Autodesk Inventor part; units mm, degrees
ref_plane "YZ Plane" through (0, 0, 0) normal (1, 0, 0) x (0, 1, 0)
ref_plane "XZ Plane" through (0, 0, 0) normal (0, 1, 0) x (-1, 0, 0)
ref_plane "XY Plane" through (0, 0, 0) normal (0, 0, 1) x (1, 0, 0)
sketch "Sketch1" plane through (0, 0, 0) normal (0, 0, 1) x (1, 0, 0)
  line L0 (0, 0) -> (33, 0)
  line L1 (33, 0) -> (33, 28)
  line L2 (33, 28) -> (0, 28)
  line L3 (0, 28) -> (0, 0)
  circle A0 centre (16.5, 14) radius 4
  circle A1 centre (16.5, 23.5) radius 1.5
  circle A2 centre (9, 5) radius 1.5
  circle A3 centre (24, 5) radius 1.5
  dimension "d0" = 33
  dimension "d1" = 28
  dimension "d2" = 8
  dimension "d3" = 14
  dimension "d4" = 16.5
  dimension "d5" = 3
  dimension "d6" = 3
  dimension "d7" = 3
  dimension "d8" = 4.5
  dimension "d9" = 0
  dimension "d10" = 15
  dimension "d11" = 5
  dimension "d12" = 9
  dimension "d13" = 5
extrude "Extrusion1" add sketch "Sketch1" along normal blind 3
sketch "Sketch2" plane through (0, 0, 3) normal (0, 0, 1) x (1, 0, 0)
  circle A0 centre (16.5, 14) radius 4
  circle A1 centre (16.5, 14) radius 5.5
  point P0 (0, 0)
  dimension "d16" = 11
extrude "Extrusion2" cut sketch "Sketch2" against normal blind 2 contours A0 | A1
fillet "Fillet1" radius 15 2 edges at (33, 28, 1.5) (0, 28, 1.5)
equation "\"d3\" = 0.5 * d1"
equation "\"d4\" = 0.5 * d0"
properties part number "Arm6" material "Aluminum 6061, Welded"
Read the model definition and answer for the solid it produces. Units are mm, in the model's axes. A direction names the side the tool comes from. Round coordinates to 2 decimals unless told otherwise and drop trailing zeros. Write each loop counter-clockwise with the first axis right and the second up, starting at its lowest first coordinate (ties: lowest second). Pieces come first, ordered by that corner, then holes. Notation, with made-up numbers: M -29,79 L 25,79 A17 cw 25,105 Z; hole C 63,21 d4. An arc over 180 degrees is marked long. Use a Markdown table: item, result.
1) Flat-ended cylindrical pins translate along their axes: pin 1 (2.5 mm diameter, centred on x = 9, y = 5, fed in from -Z); pin 2 (1 mm diameter, centred on x = 4, z = 1, fed in from +Y). Find the tip coordinate at first contact, or state that the pin passes through.
Answers follow:
| item | result |
|---|---|
| pin 1 | passes through |
| pin 2 | stops at y = 23.71 |
2) The part is cut by section B-B (y = 5). Write down the section's boundary in (x, z), plus the area to 3 significant figures.
Answers follow:
| item | result |
|---|---|
| outline | M 0,0 L 7.5,0 L 7.5,3 L 0,3 Z; M 10.5,0 L 22.5,0 L 22.5,3 L 10.5,3 Z; M 25.5,0 L 33,0 L 33,3 L 25.5,3 Z |
| area | 81.0 mm2 |
3) A tool of negligible diameter and unlimited length cuts with its end or side. For faces 4 (the cylindrical face through (4.51, 23.72, 1.52)), 5 (the cylindrical face through (15.31, 8.63, 2.01)), from which of +Z, -Z, +X, -X, +Y, -Y can it reach the whole face along a straight path? Write none if from no direction.
Answers follow:
| item | result |
|---|---|
| face 4 | +Z, -Z, -X, +Y |
| face 5 | +Z |
4) The part is cut by section C-C (z = 0.35). Write down the section's boundary in (x, y), plus the area to 3 significant figures.
Answers follow:
| item | result |
|---|---|
| outline | M 0,0 L 33,0 L 33,13 A15 ccw 18,28 L 15,28 A15 ccw 0,13 Z; hole C 9,5 d3; hole C 16.5,14 d8; hole C 16.5,23.5 d3; hole C 24,5 d3 |
| area | 756 mm2 |
5) Straight lines are drawn through the part: line 1 along Y through (x, z) = (16.5, 2.2); line 2 along Y through (x, z) = (17.5, 0.75); line 3 along X through (y, z) = (3.75, 1.45). For each, find the intervals that lie inside material, in ascending order. Write a range as [from, to].
Answers follow:
| item | result |
|---|---|
| line 1 | y = [0, 8.5], [19.5, 22], [25, 28] |
| line 2 | y = [0, 10.13], [17.87, 22.38], [24.62, 28] |
| line 3 | x = [0, 8.17], [9.83, 23.17], [24.83, 33] |
6) For a pull along X with two mould halves and no side action, classify faces 1 (the flat face through (17, 28, 1)), 2 (the cylindrical face through (12.504, 13.824, 0.493)), 3 (the flat face through (0, 7, 1)) as pulls with the +X half, pulls with the -X half, needs draft (parallel to the pull), parting line crosses it, or undercut.
Answers follow:
| item | result |
|---|---|
| face 1 | needs draft |
| face 2 | undercut |
| face 3 | pulls with the -X half |
7) The part is cut by section A-A (x = 16.5). Write down the section's boundary in (y, z).
Answers follow:
| item | result |
|---|---|
| outline | M 0,0 L 10,0 L 10,1 L 8.5,1 L 8.5,3 L 0,3 Z; M 18,0 L 22,0 L 22,3 L 19.5,3 L 19.5,1 L 18,1 Z; M 25,0 L 28,0 L 28,3 L 25,3 Z |
8) The part is cut by section D-D (y = 14). Write down the section's boundary in (x, z).
Answers follow:
| item | result |
|---|---|
| outline | M 0.03,0 L 12.5,0 L 12.5,1 L 11,1 L 11,3 L 0.03,3 Z; M 20.5,0 L 32.97,0 L 32.97,3 L 22,3 L 22,1 L 20.5,1 Z |
